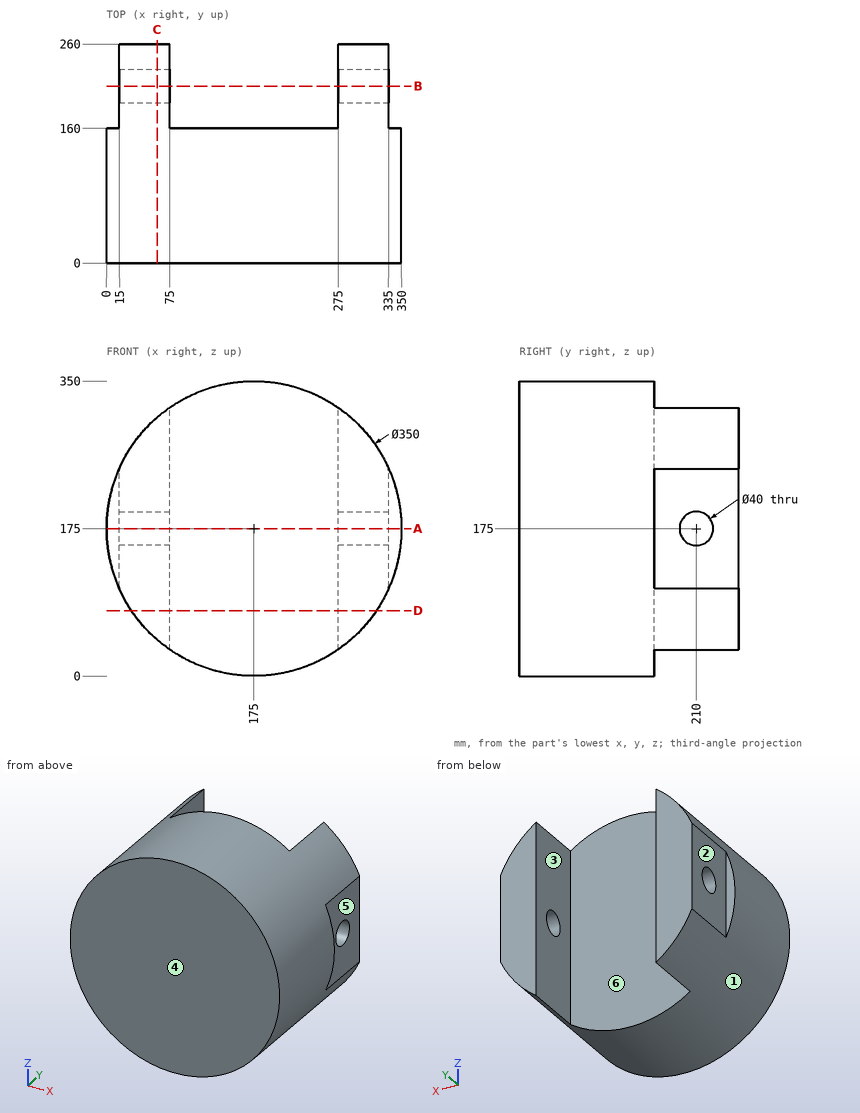
Geometry check sheet. Reference: drawing and pictorial views, mm from the part's lowest x, y, z. A direction names the side the tool comes from. Coordinates: 2 decimals unless noted, no trailing zeros. Loops run counter-clockwise (first coordinate to the right, second up) from the corner with the lowest first, then second, coordinate; pieces in that order, holes last. Notation, with made-up numbers: M 89.5,53.25 L 108.5,53.25 A18 ccw 108.5,59.25 Z; hole C 73,48.5 d4. An arc over 180 degrees is marked long. One line per item, written item: value.
1. Section check B-B on y = 210. Record the cut outline in (x, z).
Answers follow:
outline: M 15,104.11 A175 ccw 75,31.39 L 75,155 L 15,155 Z; M 15,195 L 75,195 L 75,318.61 A175 ccw 15,245.89 Z; M 275,31.39 A175 ccw 335,104.11 L 335,155 L 275,155 Z; M 275,195 L 335,195 L 335,245.89 A175 ccw 275,318.61 Z
2. Gauge pin test, flat ends, axial feed: P1, Ø1, axis at y = 99.5, z = 119, coming from the -X side; P2, Ø1, axis at y = 74.5, z = 187.5, coming from the -X side; P3, Ø12, axis at y = 225.5, z = 311.5, coming from the -X side. Record the tip position at first contact, or that the pin passes through.
Answers follow:
P1: x = 9.03
P2: x = 0.41
P3: x = 58.4
3. Material ranges on line 1 along Y through (x, z) = (288.5, 175); line 2 along Y through (x, z) = (79.5, 265); line 3 along X through (y, z) = (206, 220), recorded low to high. Write a range as from..to.
Answers follow:
line 1: 0..190, 230..260
line 2: 0..160
line 3: 15..75, 275..335
4. Set-up check for the marked faces 1 and 2: record each of +Z, -Z, +X, -X, +Y, -Y from which the full face is reachable in a straight line by a thin tool's end or side.
Answers follow:
face 1: +Y, -Y
face 2: +Z, -Z, -X, +Y
5. Mould release check, pull along X, two halves, no side actions. Record for the marked faces 3, 4, 5 and 6: pulls with the +X half, pulls with the -X half, needs draft (parallel to the pull), parting line crosses it, or undercut.
Answers follow:
face 3: undercut
face 4: needs draft
face 5: pulls with the +X half
face 6: undercut
6. Section check C-C on x = 60. Record the cut outline in (y, z), plus the area to 3 significant figures.
Answers follow:
outline: M 0,43.09 L 260,43.09 L 260,306.91 L 0,306.91 Z; hole C 210,175 d40
area: 67,300 mm^2
7. Section check D-D on z = 77.5. Record the cut outline in (x, y), plus the area to 3 significant figures.
Answers follow:
outline: M 29.68,0 L 320.32,0 L 320.32,260 L 275,260 L 275,160 L 75,160 L 75,260 L 29.68,260 Z
area: 55,600 mm^2
8. Section check A-A on z = 175. Record the cut outline in (x, y), plus the area to 3 significant figures.
Answers follow:
outline: M 0,0 L 350,0 L 350,160 L 335,160 L 335,190 L 275,190 L 275,160 L 75,160 L 75,190 L 15,190 L 15,160 L 0,160 Z; M 15,230 L 75,230 L 75,260 L 15,260 Z; M 275,230 L 335,230 L 335,260 L 275,260 Z
area: 63,200 mm^2
